from build123d import *

# Parameters (mm, degrees)
BOSS_EXTRUDE1_DEPTH     = 3
CUT_EXTRUDE1_DEPTH      = 18.219175358
CUT_EXTRUDE1_DEPTH_BACK = 18.219175358
SKETCH10_R              = 3
SKETCH11_R              = 1.5
CUT_EXTRUDE2_DEPTH      = 10
FILLET1_R               = 3
CUT_EXTRUDE3_START      = -2
SKETCH12_R              = 4.5
CUT_EXTRUDE3_DEPTH      = 10


with BuildPart() as part:
    # Sketch1 → Boss-Extrude1 (new, symmetric)
    with BuildSketch(Plane.XY):
        with BuildLine():
            Line((3.354101966, -3), (15.5, -3))
            Line((15.5, -3), (15.5, 3))
            Line((15.5, 3), (3.354101966, 3))
            ThreePointArc((3.354101966, 3), (-4.5, 0), (3.354101966, -3))
        make_face()
    extrude(amount=BOSS_EXTRUDE1_DEPTH, both=True)

    # Sketch10 → Cut-Extrude1 (cut, two sides: drawn at the far end of the back side and taken through both)
    with BuildSketch(Plane.XY.offset(3).offset(-CUT_EXTRUDE1_DEPTH_BACK)):
        Circle(SKETCH10_R)
    extrude(amount=CUT_EXTRUDE1_DEPTH + CUT_EXTRUDE1_DEPTH_BACK, mode=Mode.SUBTRACT)

    # Sketch11 → Cut-Extrude2 (cut)
    with BuildSketch(Plane(origin=(15.5, 0, 0), x_dir=(0, 0, -1), z_dir=(1, 0, 0))):
        Circle(SKETCH11_R)
    extrude(amount=-CUT_EXTRUDE2_DEPTH, mode=Mode.SUBTRACT)

    # Fillet1
    fillet1_edges = [part.edges().sort_by_distance(p)[0] for p in [
        (9.427050983, -3, 3),
        (9.427050983, -3, -3),
        (9.427050983, 3, -3),
        (9.427050983, 3, 3),
    ]]
    fillet(fillet1_edges, radius=FILLET1_R - 0.0001)  # a hair under: the kernel refuses the full size

    # Sketch12 → Cut-Extrude3 (cut)
    with BuildSketch(Plane.XY.offset(CUT_EXTRUDE3_START)):
        Circle(SKETCH12_R)
    cut_extrude3 = extrude(amount=-CUT_EXTRUDE3_DEPTH, mode=Mode.SUBTRACT)

    # Mirror1: Cut-Extrude3 across plane
    add(cut_extrude3.mirror(Plane.XY), mode=Mode.SUBTRACT)


solid = part.part
Geometry: final body of the model. Coordinates: model frame, mm. A direction names the side the tool comes from. Give positions to 0.01 mm unless a question says otherwise; leave off trailing zeros. Loops run counter-clockwise (first coordinate to the right, second up) from the corner with the lowest first, then second, coordinate; pieces in that order, holes last. Notation, with made-up numbers: M 77.25,22.25 L 87.25,22.25 A29 ccw 87.25,45.25 Z; hole C 38.5,80 d7. An arc over 180 degrees is marked long. Put each result on its own line as item: value. Start each with the question number.
1) Contact query for flat-ended pins moving along their axis: pin 1 (0.9 mm diameter, centred on y = 0.5, z = 0.5, fed in from +X); pin 2 (4 mm diameter, centred on x = 4, y = 2.5, fed in from -Z); pin 3 (1 mm diameter, centred on x = 9.5, z = 1.5, fed in from -Y). Output: stop coordinate, or through.
2) Pull-direction query (Y, two-part tool) for faces 1 (the cylindrical face through (9.34, 2.1, -2.14)), 2 (the cylindrical face through (10.57, 0.07, 1.5)), 3 (the cylindrical face through (9.51, -2.14, -2.1)); classes: pulls with the +Y half, pulls with the -Y half, needs draft (parallel to the pull), parting line crosses it, or undercut.
3) Cut plane A-A (x = 0). Output: boundary loops of the cut face in (y, z).
4) Cut plane B-B (y = -2). Output: boundary loops of the cut face in (x, z).
5) Access query for faces 4 (the flat face through (1, -3, -2)), 5 (the cylindrical face through (9.51, -2.14, 2.1)), 6 (the cylindrical face through (4.5, 0, 2.4)), 7 (the cylindrical face through (9.34, 2.1, 2.14)), 8 (the flat face through (5.5, 0, 0)). Directions: +Z, -Z, +X, -X, +Y, -Y. A direction counts if a zero-diameter tool reaches every point of the face in a straight line with its end or side. Return the directions, or none.
6) Ray query, line 1 along X through (y, z) = (0, -1.1); line 2 along Y through (x, z) = (9, 0); line 3 along Y through (x, z) = (0, 0.95). Return the intervals inside material, ascending.
7) Cut plane C-C (z = -1). Output: boundary loops of the cut face in (x, y).
Verdict:
1. pin 1: x = 5.5
1. pin 2: z = -2.95
1. pin 3: y = -2.83
2. face 1: pulls with the +Y half
2. face 2: undercut
2. face 3: pulls with the -Y half
3. outline: M -4.5,-2 L -3,-2 L -3,2 L -4.5,2 Z; M 3,-2 L 4.5,-2 L 4.5,2 L 3,2 Z
4. outline: M -4.03,-2 L -2.24,-2 L -2.24,2 L -4.03,2 Z; M 2.24,-2 L 4.03,-2 L 4.03,-2.24 L 15.5,-2.24 L 15.5,2.24 L 4.03,2.24 L 4.03,2 L 2.24,2 Z
5. face 4: -Z, -X
5. face 5: +Z, +X, -Y
5. face 6: +Z, -X
5. face 7: +Z, +X, +Y
5. face 8: +X
6. line 1: -4.5 to -3, 3 to 5.5
6. line 2: -3 to -1.5, 1.5 to 3
6. line 3: -4.5 to -3, 3 to 4.5
7. outline: M 3.5,-2.83 L 15.5,-2.83 L 15.5,-1.12 L 5.5,-1.12 L 5.5,1.12 L 15.5,1.12 L 15.5,2.83 L 3.5,2.83 A4.5 ccw long Z; hole C 0,0 d6
